The figure shows three views and two pictorial views of one solid part (mm, origin at its lowest corner). Answer the questions. A direction names the side the tool comes from. Coordinates: 2 decimals unless noted, no trailing zeros. Loops run counter-clockwise (first coordinate to the right, second up) from the corner with the lowest first, then second, coordinate; pieces in that order, holes last. Notation, with made-up numbers: (45, -4) - (92, -4) arc R22 ccw to (92, 4) - close; hole circle Ø6 at (6.25, 17.25). An arc over 180 degrees is marked (long way). Return JSON: item names as keys, results as strings. Group by question number.
1. Find the intervals of material crossed by line 1 along Z through (x, y) = (6, 4.2); line 2 along Y through (x, z) = (1, 14); line 3 along Z through (x, y) = (9.25, 1.35), in increasing order.
2. This flat-tipped pin is pushed along its axis until it touches: P1, Ø2.5, axis at x = 12.5, z = 17, coming from the +Y side. Where does it stop, or does it pass through?
3. Which of the six approach directions +Z, -Z, +X, -X, +Y, -Y give full straight-line access (tool end or side, diameter ignored) to the marked faces 1 and 2?
4. Section B-B (z = 17.75) is taken. Write down the section's boundary in (x, y), and give its area (3 significant figures).
5. Section C-C (x = 4) is taken. Write down the section's boundary in (y, z), and give its area (3 significant figures).
6. Section A-A (x = 10.75) is taken. Write down the section's boundary in (y, z), and give its area (3 significant figures).
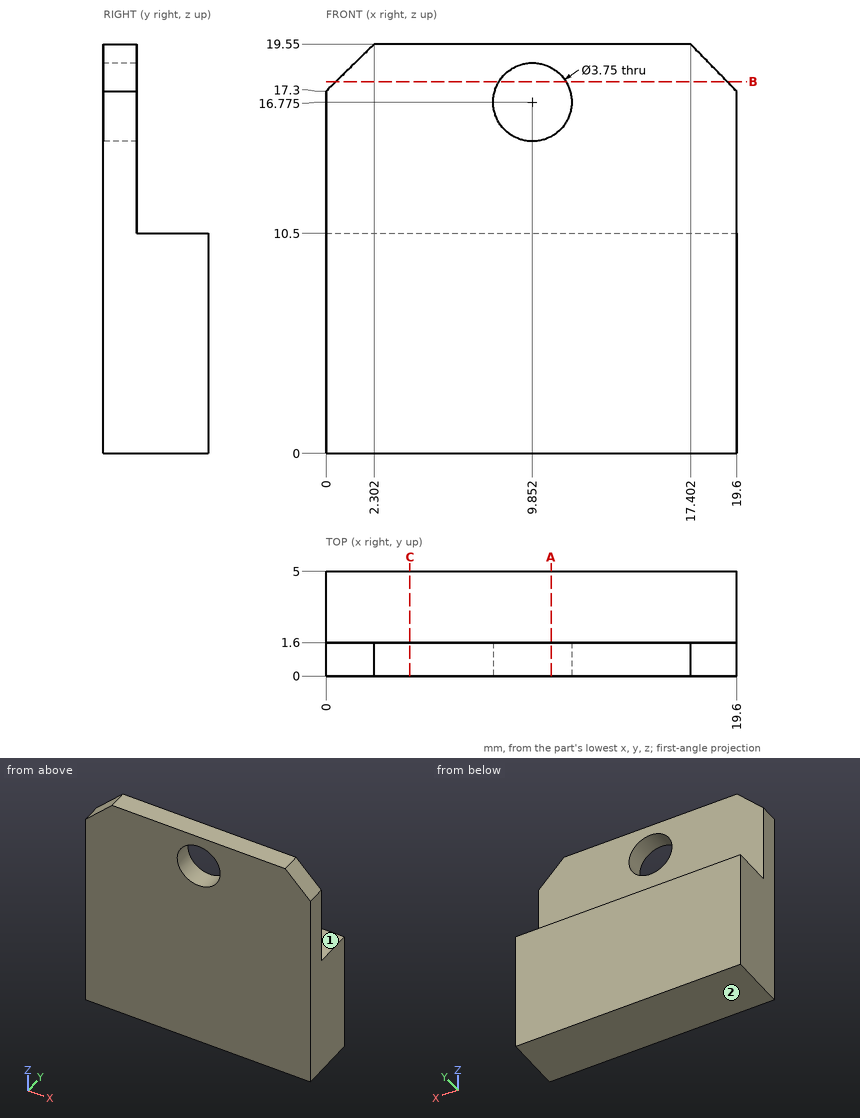
The answers:
{
 "1": {"line 1": "z = 0 to 10.5", "line 2": "y = 0 to 1.6", "line 3": "z = 0 to 15, 18.55 to 19.55"},
 "2": {"P1": "stops at y = 1.6"},
 "3": {"face 1": "+Z, +X, -X, +Y", "face 2": "-Z, +X, -X, +Y, -Y"},
 "4": {"outline": "(0.46, 0) - (8.25, 0) - (8.25, 1.6) - (0.46, 1.6) - close; (11.45, 0) - (19.16, 0) - (19.16, 1.6) - (11.45, 1.6) - close", "area": "24.8 mm2"},
 "5": {"outline": "(0, 0) - (5, 0) - (5, 10.5) - (1.6, 10.5) - (1.6, 19.55) - (0, 19.55) - close", "area": "67.0 mm2"},
 "6": {"outline": "(0, 0) - (5, 0) - (5, 10.5) - (1.6, 10.5) - (1.6, 15.13) - (0, 15.13) - close; (0, 18.42) - (1.6, 18.42) - (1.6, 19.55) - (0, 19.55) - close", "area": "61.7 mm2"}
}
